Print and shaded views of the part. All mm, measured from the part's lowest x, y and z. A direction names the side the tool comes from. Coordinates: 2 decimals unless noted, no trailing zeros. Order: outer loops, then holes, each group sorted by start corner. A loop starts at its lowest first (then second) coordinate and runs counter-clockwise, first axis right, second up. Notation, with made-up numbers: M 76.25,88 L 95.25,88 A21 cw 95.25,123 Z; hole C 82.25,14.25 d8. An arc over 180 degrees is marked long. Use a Markdown table: item, result. Add a question column.
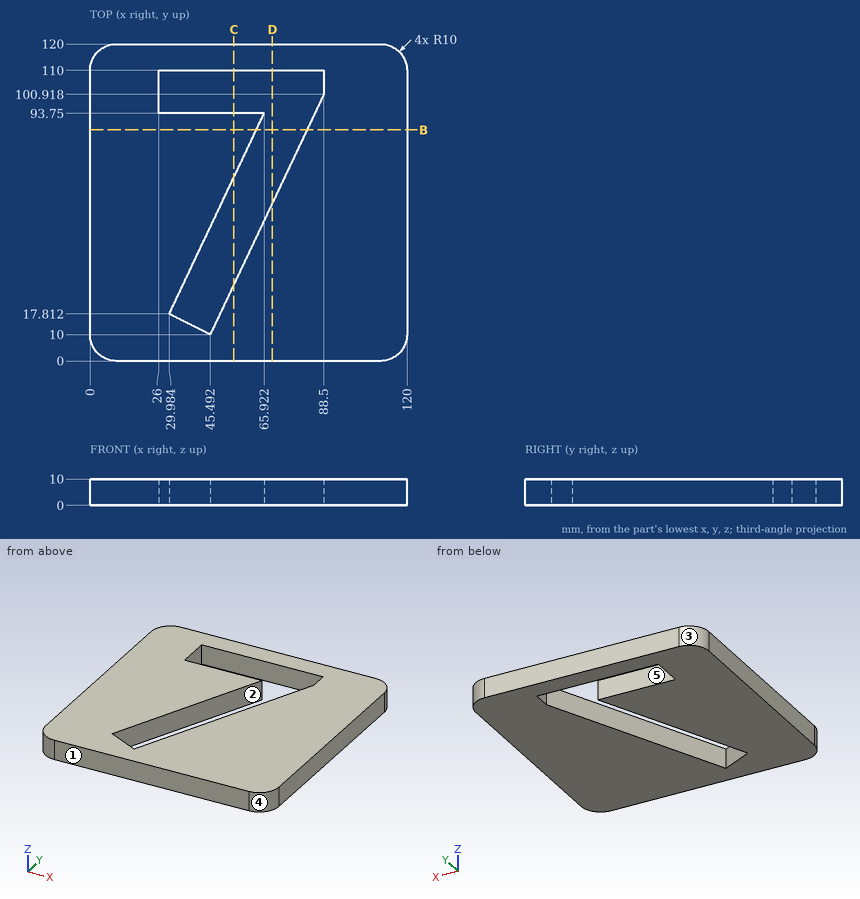
(1) Which spindle directions (+Z, -Z, +X, -X, +Y, -Y) get a long thin tool onto all of the face, cutting with end or side? Do the marked faces 4 and 5. Say none if no direction does.
(2) Mould opens along X. For the marked faces 1, 2 and 3 say: released by +X, released by -X, zero draft, split by the parting line, or undercut.
(3) Slice it at C-C on x = 54.5. State how many separate pieces and enclosed holes the cut face has, and give its area (3 significant figures).
(4) Slice it at B-B on y = 87.5. Give the cut face in (x, z) (1 decimal), and give its area (3 significant figures).
(5) Slice it at D-D on x = 69. Give the cut face in (y, z) (1 decimal).
(6) Drill centre lines: line 1 along X through (y, z) = (51.5, 7.25) (1 decimal); line 2 along X through (y, z) = (37.5, 4.75); line 3 along Y through (x, z) = (74, 8.25) (1 decimal). Where is each one in solid material? Low to high. Write a range as from..to.
(7) Drop a flat-ended pin along its axis: P1, Ø1, axis at x = 32, y = 38, coming from the -Z side. Give the stop position or say it passes through.
Solutions:
| question | item | result |
|---|---|---|
| 1 | face 4 | +Z, -Z, +X, -Y |
| 1 | face 5 | +Z, -Z |
| 2 | face 1 | zero draft |
| 2 | face 2 | undercut |
| 2 | face 3 | released by -X |
| 3 | separate pieces | 3 |
| 3 | enclosed holes | 0 |
| 3 | area | 632 mm² |
| 4 | outline | M 0,0 L 63,0 L 63,10 L 0,10 Z; M 82.2,0 L 120,0 L 120,10 L 82.2,10 Z |
| 4 | area | 1,010 mm² |
| 5 | outline | M 0,0 L 59.7,0 L 59.7,10 L 0,10 Z; M 110,0 L 120,0 L 120,10 L 110,10 Z |
| 6 | line 1 | 0..45.9, 65.1..120 |
| 6 | line 2 | 0..39.3, 58.5..120 |
| 6 | line 3 | 0..70.3, 110..120 |
| 7 | P1 | z = 0 |
